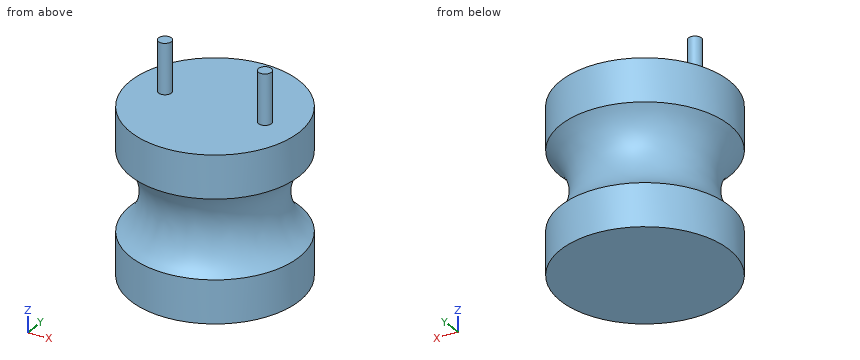
```python
from build123d import *

# Parameters (mm, degrees)
SKETCH_2_R      = 0.45
EXTRUDE_1_DEPTH = 3.5


with BuildPart() as part:
    # Эскиз1 → Повернуть1 (revolve)
    with BuildSketch(Plane(origin=(0, 0, 0), x_dir=(1, 0, 0), z_dir=(0, 1, 0)), mode=Mode.PRIVATE) as revolve_1_sk:
        with BuildLine():
            Line((0, 0), (0, 11.5))
            Line((0, 11.5), (-5.9, 11.5))
            Line((-5.9, 11.5), (-5.9, 8.5))
            ThreePointArc((-5.9, 8.5), (-4.5, 5.75), (-5.9, 3))
            Line((-5.9, 3), (-5.9, 0))
            Line((-5.9, 0), (0, 0))
        make_face()
    revolve(revolve_1_sk.sketch.rotate(Axis((0, 0, 0), (0, 0, -1)), 180), axis=Axis((0, 0, 0), (0, 0, -1)))

    # Эскиз2 → Бобышка-Вытянуть1 (add)
    with BuildSketch(Plane.XY):
        with Locations(Location((-3.5, 0, 0), (0, 0, 180))):
            Circle(SKETCH_2_R)
        with Locations(Location((3.5, 0, 0), (0, 0, 180))):
            Circle(SKETCH_2_R)
    extrude(amount=EXTRUDE_1_DEPTH)


solid = part.part
```
Design review of the part built by this model. Coordinates are the model's own, in mm. Coordinates: 2 decimals unless noted, no trailing zeros. Order: outer loops, then holes, each group sorted by start corner. A loop starts at its lowest first (then second) coordinate and runs counter-clockwise, first axis right, second up. Notation, with made-up numbers: (31, 73) - (80, 73) arc R34 cw to (80, 108) - close; hole circle Ø11 at (-24, 5.5). An arc over 180 degrees is marked (long way). One line per question, with ' | ' between items.
Q1. Consider section C-C, the plane z = 1.75. Give the boundary of the cut face in (x, y), then the cut area to 3 significant figures.
Answer key:
outline: circle Ø0.9 at (-3.5, 0); circle Ø0.9 at (3.5, 0) | area: 1.27 mm2
Q2. To check wall thickness, follow line 1 along Z through (x, y) = (1, -0.75); line 2 along Z through (x, y) = (-5.25, 1.5); line 3 along Z through (x, y) = (-0.25, 4.75). State the ranges of each line that lie inside material, in increasing order.
Answer key:
line 1: z = -11.5 to 0 | line 2: z = -11.5 to -8.12, -3.38 to 0 | line 3: z = -11.5 to -7.05, -4.45 to 0
Q3. Clearance check with flat-ended pins moving along their axes: pin 1 Ø3 at (x, z) = (4.5, 0) entering from +Y; pin 2 Ø2 at (y, z) = (-0.5, -5.5) entering from +X; pin 3 Ø3 at (x, z) = (-4.5, -8) entering from +Y. State where each tip first meets the part, or that it passes through.
Answer key:
pin 1: stops at y = 5.08 | pin 2: stops at x = 4.72 | pin 3: stops at y = 5.03
Q4. Consider section D-D, the plane z = -1.75. Give the boundary of the cut face in (x, y), then the cut area to 3 significant figures.
Answer key:
outline: circle Ø11.8 at (0, 0) | area: 109 mm2
Q5. Consider section A-A, the plane y = 0. Give the boundary of the cut face in (x, z).
Answer key:
outline: (-5.9, -11.5) - (5.9, -11.5) - (5.9, -8.5) arc R3.4 cw to (5.9, -3) - (5.9, 0) - (3.95, 0) - (3.95, 3.5) - (3.05, 3.5) - (3.05, 0) - (-3.05, 0) - (-3.05, 3.5) - (-3.95, 3.5) - (-3.95, 0) - (-5.9, 0) - (-5.9, -3) arc R3.4 cw to (-5.9, -8.5) - close
Q6. Consider section B-B, the plane x = 0. Give the boundary of the cut face in (y, z), then the cut area to 3 significant figures.
Answer key:
outline: (-5.9, -11.5) - (5.9, -11.5) - (5.9, -8.5) arc R3.4 cw to (5.9, -3) - (5.9, 0) - (-5.9, 0) - (-5.9, -3) arc R3.4 cw to (-5.9, -8.5) - close | area: 125 mm2
